Design review of the part built by this model. Coordinates are the model's own, in mm. Face numbers are marked on the shaded views. A direction names the side the tool comes from. Give positions to 0.01 mm unless a question says otherwise; leave off trailing zeros. Loops run counter-clockwise (first coordinate to the right, second up) from the corner with the lowest first, then second, coordinate; pieces in that order, holes last. Notation, with made-up numbers: (34, -14) -> (50, -14) arc R9 cw to (50, -6) -> close; hole circle Ø8 at (-31, 3). An arc over 180 degrees is marked (long way). Use CSV: the item, a comma, the result in double quotes. Start each with the question number.
Item 1: We need section A-A (z = -16). State the section outline as (x, y) points, plus the area to 3 significant figures.
Item 2: Clearance check with flat-ended pins moving along their axes: pin 1 (1 mm diameter, centred on x = 30, y = 2, fed in from -Z); pin 2 (3 mm diameter, centred on x = 17.5, z = -4.5, fed in from +Y); pin 3 (6.5 mm diameter, centred on y = 16, z = -16, fed in from -X). State where each tip first meets the part, or that it passes through.
Item 3: We need section B-B (x = 11). State the section outline as (y, z) points, plus the area to 3 significant figures.
Item 4: We need section D-D (x = 17.5). State the section outline as (y, z) points, plus the area to 3 significant figures.
Item 5: We need section C-C (y = 16). State the section outline as (x, z) points, plus the area to 3 significant figures.
Item 6: For the marked faces 1 and 2, list the 3-axis set-ups (+Z, -Z, +X, -X, +Y, -Y) from which the entire face can be reached by the end or side of a thin tool; tool diameter is ignored.
Item 7: The part is to be moulded in two halves that separate along Y. For the marked faces 3, 4 and 5, say which applies: +Y half, -Y half, draft (parallel to the pull), parting line (faces both ways), or undercut.
Item 8: Wall thickness on line 1 along X through (y, z) = (36, -3.5); line 2 along Y through (x, z) = (28.15, -16); line 3 along Z through (x, y) = (26, 7): over which ranges is each line inside the solid? List them lowest first. Write a range as from..to.
from build123d import *

# Parameters (mm, degrees)
SALIENTE_EXTRUIR1_DEPTH = 28
CROQUIS2_W              = 34
CROQUIS2_H              = 34
SALIENTE_EXTRUIR2_DEPTH = 7
REDONDEO1_R             = 5
CROQUIS3_R              = 3.5
CORTAR_EXTRUIR1_DEPTH   = 5
CROQUIS4_R              = 2
CORTAR_EXTRUIR2_DEPTH   = 5
CROQUIS5_R              = 3.5
CORTAR_EXTRUIR3_DEPTH   = 5
CROQUIS6_R              = 2
CORTAR_EXTRUIR4_DEPTH   = 5
REDONDEO2_R             = 5
SALIENTE_EXTRUIR3_START = 10
SALIENTE_EXTRUIR3_DEPTH = 10


with BuildPart() as part:
    # Croquis1 → Saliente-Extruir1 (new body)
    with BuildSketch(Plane(origin=(0, 0, 0), x_dir=(1, 0, 0), z_dir=(0, 1, 0))):
        Polygon((0, 0), (27, 0), (27, 27), (34, 27), (34, -7), (0, -7), align=None)
    extrude(amount=SALIENTE_EXTRUIR1_DEPTH)

    # Croquis2 → Saliente-Extruir2 (add)
    with BuildSketch(Plane(origin=(0, 0, 0), x_dir=(-1, 0, 0), z_dir=(0, -1, 0))):
        with Locations((-17, 10)):
            Rectangle(CROQUIS2_W, CROQUIS2_H)
    extrude(amount=SALIENTE_EXTRUIR2_DEPTH)

    # Redondeo1
    redondeo1_edges = [part.edges().sort_by_distance(p)[0] for p in [
        (34, 10.5, -27),
        (34, 10.5, 7),
        (0, 10.5, 7),
        (34, -7, -10),
        (17, -7, 7),
    ]]
    fillet(redondeo1_edges, radius=REDONDEO1_R)

    # Croquis3 → Cortar-Extruir1 (cut)
    with BuildSketch(Plane(origin=(34, 0, 0), x_dir=(0, 0, -1), z_dir=(1, 0, 0))):
        with Locations((16, 16)):
            Circle(CROQUIS3_R)
    extrude(amount=-CORTAR_EXTRUIR1_DEPTH, mode=Mode.SUBTRACT)

    # Croquis4 → Cortar-Extruir2 (cut)
    with BuildSketch(Plane(origin=(29, 0, 0), x_dir=(0, 0, -1), z_dir=(1, 0, 0))):
        with Locations((16, 16)):
            Circle(CROQUIS4_R)
    extrude(amount=-CORTAR_EXTRUIR2_DEPTH, mode=Mode.SUBTRACT)

    # Croquis5 → Cortar-Extruir3 (cut)
    with BuildSketch(Plane.XY.offset(7)):
        with Locations((11, 16)):
            Circle(CROQUIS5_R)
    extrude(amount=-CORTAR_EXTRUIR3_DEPTH, mode=Mode.SUBTRACT)

    # Croquis6 → Cortar-Extruir4 (cut)
    with BuildSketch(Plane.XY.offset(2)):
        with Locations((11, 16)):
            Circle(CROQUIS6_R)
    extrude(amount=-CORTAR_EXTRUIR4_DEPTH, mode=Mode.SUBTRACT)

    # Redondeo2
    # the kernel refuses this fillet: 5 mm, written as the material it takes off along each edge
    with BuildSketch(Plane(origin=(29, -2, -22), x_dir=(0, -1, 0), z_dir=(0, 0, -1))) as redondeo2_piece_1_section:
        Polygon((0, 0), (REDONDEO2_R, 0), (REDONDEO2_R, -REDONDEO2_R), (0, -REDONDEO2_R), align=None)
    redondeo2_piece_1 = extrude(amount=REDONDEO2_R, mode=Mode.PRIVATE)
    redondeo2_piece_1 = redondeo2_piece_1 - Plane(origin=(29, -2, -22), x_dir=(-0.7071067811865475, 0.7071067811865475, 0), z_dir=(0, 0, -1)) * Sphere(REDONDEO2_R, mode=Mode.PRIVATE)
    add(redondeo2_piece_1, mode=Mode.SUBTRACT)
    with BuildSketch(Plane(origin=(5, -2, 2), x_dir=(0, -1, 0), z_dir=(-1, 0, 0))) as redondeo2_piece_2_section:
        Polygon((0, 0), (REDONDEO2_R, 0), (REDONDEO2_R, REDONDEO2_R), (0, REDONDEO2_R), align=None)
    redondeo2_piece_2 = extrude(amount=REDONDEO2_R, mode=Mode.PRIVATE)
    redondeo2_piece_2 = redondeo2_piece_2 - Plane(origin=(5, -2, 2), x_dir=(0, 0.7071067811865475, -0.7071067811865475), z_dir=(-1, 0, 0)) * Sphere(REDONDEO2_R, mode=Mode.PRIVATE)
    add(redondeo2_piece_2, mode=Mode.SUBTRACT)
    with BuildSketch(Plane(origin=(-12.5, -7, -27), x_dir=(0, 1, 0), z_dir=(1, 0, 0)), Plane(origin=(0, -7, 2), x_dir=(0, 1, 0), z_dir=(0, 0, -1))) as redondeo2_piece_3:
        with BuildLine():
            CenterArc((REDONDEO2_R, REDONDEO2_R), REDONDEO2_R, 180, 90)
            Line((0, REDONDEO2_R), (0, 0))
            Line((0, 0), (REDONDEO2_R, 0))
        make_face()
    extrude(amount=41.5, mode=Mode.SUBTRACT)

    # Croquis7 → Saliente-Extruir3 (add)
    with BuildSketch(Plane(origin=(0, 28, 0), x_dir=(1, 0, 0), z_dir=(0, 1, 0)).offset(SALIENTE_EXTRUIR3_START)):
        with BuildLine():
            Line((34, -2), (34, 22))
            ThreePointArc((34, 22), (32.535533906, 25.535533906), (29, 27))
            Line((29, 27), (27, 27))
            Line((27, 27), (27, 0))
            Line((27, 0), (0, 0))
            Line((0, 0), (0, -2))
            ThreePointArc((0, -2), (1.464466094, -5.535533906), (5, -7))
            Line((5, -7), (29, -7))
            ThreePointArc((29, -7), (32.535533906, -5.535533906), (34, -2))
        make_face()
    extrude(amount=-SALIENTE_EXTRUIR3_DEPTH)


solid = part.part
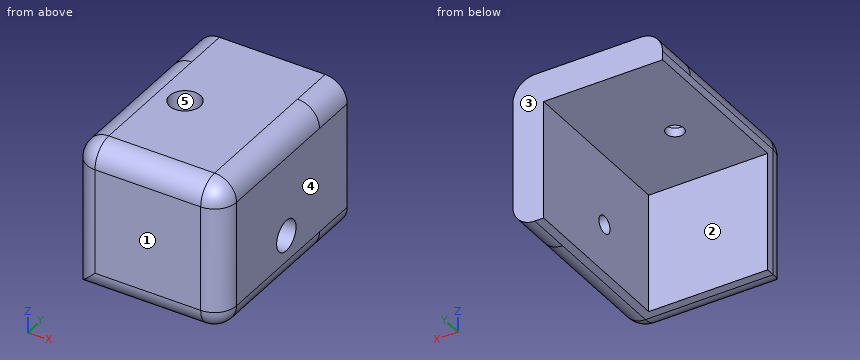
Results found:
1,outline,"(0, -2) arc R5 ccw to (5, -7) -> (29, -7) arc R5 ccw to (34, -2) -> (34, 12.5) -> (29, 12.5) -> (29, 14) -> (27, 14) -> (27, 0) -> (0, 0) -> close; (27, 18) -> (29, 18) -> (29, 19.5) -> (34, 19.5) -> (34, 38) -> (27, 38) -> close"
1,area,"450 mm²"
2,pin 1,"z = -26.97"
2,pin 2,"y = 0"
2,pin 3,"x = 27"
3,outline,"(-7, -22) arc R5 ccw to (-2, -27) -> (0, -27) -> (0, 0) -> (14, 0) -> (14, 2) -> (12.5, 2) -> (12.5, 7) -> (-2, 7) arc R5 ccw to (-7, 2) -> close; (18, 0) -> (38, 0) -> (38, 7) -> (19.5, 7) -> (19.5, 2) -> (18, 2) -> close"
3,area,"450 mm²"
4,outline,"(-7, -22) arc R5 ccw to (-2, -27) -> (0, -27) -> (0, 0) -> (38, 0) -> (38, 7) -> (-2, 7) arc R5 ccw to (-7, 2) -> close"
4,area,"493 mm²"
5,outline,"(0, 0) -> (9, 0) -> (9, 2) -> (7.5, 2) -> (7.5, 7) -> (5, 7) arc R5 ccw to (0, 2) -> close; (13, 0) -> (27, 0) -> (27, -14) -> (29, -14) -> (29, -12.5) -> (34, -12.5) -> (34, 2) arc R5 ccw to (29, 7) -> (14.5, 7) -> (14.5, 2) -> (13, 2) -> close; (27, -27) -> (29, -27) arc R5 ccw to (34, -22) -> (34, -19.5) -> (29, -19.5) -> (29, -18) -> (27, -18) -> close"
5,area,"325 mm²"
6,face 1,"+Z, -Z, +X, -X, -Y"
6,face 2,"-Z, -X, +Y"
7,face 3,"+Y half"
7,face 4,"draft"
7,face 5,"undercut"
8,line 1,"27..34"
8,line 2,"-7..14, 18..38"
8,line 3,"0..7"
